Work out the finished part from the listing and answer in its coordinate system (mm). Face numbers are marked on the shaded views. A direction names the side the tool comes from. Round coordinates to 2 decimals unless told otherwise and drop trailing zeros. Order: outer loops, then holes, each group sorted by start corner. A loop starts at its lowest first (then second) coordinate and runs counter-clockwise, first axis right, second up. Notation, with made-up numbers: M -23,-7 L 17,-7 A21 cw 17,16 Z; hole C 52,-28 d1. An arc over 180 degrees is marked long. Return JSON: item names as keys, results as strings.
Solid Edge part; units mm, degrees
sketch "Sketch1" plane through (0, 0, 0) normal (0, -1, 0) x (1, 0, 0)
  line L0 (0, -10) -> (1.5, -10)
  line L1 (1.5, -10) -> (1.5, -0.601)
  line L2 (1.5, -0.601) -> (1.3375, -0.101)
  line L3 (1.3375, -0.101) -> (1.3375, 0)
  line L4 (1.3375, 0) -> (2.8, 0)
  line L5 (2.8, 0) -> (2.6425, 1.8)
  line L6 (2.6425, 1.8) -> (0, 1.8)
  dimension "D1" = 1.3375
  dimension "D2" = 1.5
  dimension "D3" = 2.6425
revolve "RevolvedProtrusion1" add sketch "Sketch1" angle 360 about axis through (0, 0, 6) along (0, 0, -1)
fillet "Round_1" radius 0.9 1 edges at (-2.6425, 0, 1.8)
sketch "Sketch2" plane through (0, 0, 0) normal (0, -1, 0) x (1, 0, 0)
  line L0 (-0.4, 1.8) -> (-0.4, 1.1)
  line L1 (-0.4, 1.1) -> (0.4, 1.1)
  line L2 (0.4, 1.1) -> (0.4, 1.8)
  line L3 (0.4, 1.8) -> (-0.4, 1.8)
  dimension "D1" = 0.4
  dimension "D2" = 0.4
extrude "ExtrudedCutout_1" cut sketch "Sketch2" along normal mid plane 5.6
cosmetic_thread "Thread_1" thread depth 9.399
fillet "Round_2" radius 0.1 1 edges at (-1.3375, 0, 0)
chamfer "Chamfer_1" distance 0.0012 angle 30 1 edges at (-1.5, 0, -10) measured on face at (1.03, 0.97, -10)
properties material "Steel"
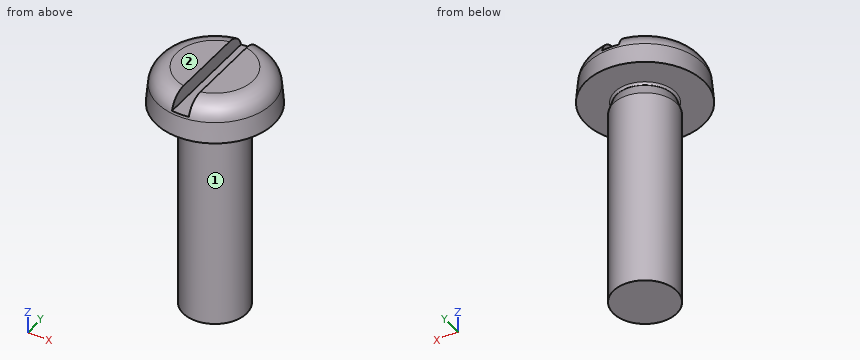
Item 1: Consider line 1 along X through (y, z) = (-0.05, -2); line 2 along Y through (x, z) = (-1.7, 0.5); line 3 along X through (y, z) = (2.1, 1). Determine where each line is inside the solid, lowest interval first. Write a range as [from, to].
Output:
{"line 1": "x = [-1.5, 1.5]", "line 2": "y = [-2.17, 2.17]", "line 3": "x = [-1.72, 1.72]"}
Item 2: Find section C-C (z = -0.75). Determine the outline of the cut face in (x, y).
Output:
{"outline": "C 0,0 d3"}
Item 3: Each of these flat-tipped pins is pushed along its axis until it touches: pin 1 (1 mm diameter, centred on y = -0.5, z = -3, fed in from +X); pin 2 (0.6 mm diameter, centred on y = -1, z = 1.5, fed in from -X); pin 3 (1 mm diameter, centred on x = -0.5, z = -4, fed in from +Y). Where does it stop, or does it pass through?
Output:
{"pin 1": "stops at x = 1.5", "pin 2": "stops at x = -2.51", "pin 3": "stops at y = 1.5"}
Item 4: Which of the six approach directions +Z, -Z, +X, -X, +Y, -Y give full straight-line access (tool end or side, diameter ignored) to the marked faces 1 and 2?
Output:
{"face 1": "-Z", "face 2": "+Z, +X, -X, +Y, -Y"}
